from build123d import *

# Parameters (mm, degrees)
F2_R     = 19.05
F3_DEPTH = 25.4


with BuildPart() as f1:
    # F0 (on Right) → F1 (revolve)
    with BuildSketch(Plane.YZ):
        Polygon((-25.4, 16.811958), (0, 16.811958), (0, 26.336958), (0, 28.782088), (-6.35, 28.782088), (-6.35, 35.861958), (-25.4, 35.861958), align=None)
        Polygon((0, 26.336958), (0, 16.811958), (25.4, 16.811958), (25.4, 35.861958), (6.35, 35.861958), (6.35, 105.711958), (12.7, 105.711958), (12.7, 131.111958), (-12.7, 131.111958), (-12.7, 105.711958), (-6.35, 105.711958), (-6.35, 35.861958), (-6.35, 28.782088), (0, 28.782088), align=None)
    revolve(axis=Axis((0, 18.4531, 0), (0, 1, 0)))

    # F2 (on face) → F3 (cut)
    with BuildSketch(Plane.XZ.offset(6.35)):
        with BuildLine():
            ThreePointArc((19.05, 69.047159), (-13.470384, 82.517543), (0, 49.997159))
            ThreePointArc((0, 49.997159), (13.470384, 55.576775), (19.05, 69.047159))
        make_face()
        with Locations((69.047159, 0)):
            Circle(F2_R)
        with Locations((0, -69.047159)):
            Circle(F2_R)
        with Locations((-69.047159, 0)):
            Circle(F2_R)
    extrude(amount=-F3_DEPTH, mode=Mode.SUBTRACT)


solid = f1.part
Model file for the job. Use its own axes, mm. A direction names the side the tool comes from. Round coordinates to 2 decimals unless told otherwise and drop trailing zeros. Order: outer loops, then holes, each group sorted by start corner. A loop starts at its lowest first (then second) coordinate and runs counter-clockwise, first axis right, second up.
(1) Pin check, flat tips, straight feed: pin 1 (8 mm diameter, centred on y = -12, z = -79, fed in from +X); pin 2 (8 mm diameter, centred on x = 14.5, z = -42, fed in from -Y); pin 3 (1.5 mm diameter, centred on x = 92, y = 12, fed in from -Z); pin 4 (12 mm diameter, centred on x = 24.5, z = 27, fed in from -Y). Stop position of each tip, or through.
(2) Band-saw the part on C-C (y = 2). List the corners of the cut face in (x, z).
(3) Band-saw the part on D-D (z = 84.5). List the corners of the cut face in (x, y).
(4) Band-saw the part on B-B (x = 85). List the corners of the cut face in (y, z), then the cut area to 3 significant figures.
(5) 3-axis set-ups, long thin cutter, end or side, ignore diameter. For faces 1 (the face through (1, 6.35, -46)), 2 (the face through (35.557, -16.008, -4.669)), 3 (the face through (5.05, 0.356, 16.036)): which of +Z, -Z, +X, -X, +Y, -Y reach the whole face in a straight line?
(6) Drill centre lines: line 1 (X direction, y = 11.5, z = 1); line 2 (Z direction, x = -10, y = 9); line 3 (X direction, y = 11.25, z = 0). Where is each one in solid material? Low to high.
(7) Band-saw the part on A-A (z = 0). Give the number of separate pieces and of enclosed holes in the cut face, then the cut area to 3 significant figures.
(8) Pull direction Z, two halves, no side cores. Call faces 4 (the face through (-7.5, 25.4, -15.4)), 5 (the face through (129.996, -0.178, -17.068)), 6 (the face through (-51.45, -0.09, -7.3)): released by +Z, released by -Z, zero draft, split by the parting line, or undercut.
Verdict:
1. pin 1: stops at x = 107.54
1. pin 2: stops at y = -6.35
1. pin 3: stops at z = -94.15
1. pin 4: stops at y = -25.4
2. outline: circle Ø262.22 at (0, 0); hole circle Ø38.1 at (-69.05, 0); hole circle Ø38.1 at (0, -69.05); hole circle Ø38.1 at (0, 69.05); hole circle Ø33.62 at (0, 0); hole circle Ø38.1 at (69.05, 0)
3. outline: (-100.25, -12.7) - (-63.52, -12.7) - (-63.52, -6.35) - (-11.14, -6.35) - (-11.14, 6.35) - (-63.52, 6.35) - (-63.52, 12.7) - (-100.25, 12.7) - close; (11.14, -6.35) - (63.52, -6.35) - (63.52, -12.7) - (100.25, -12.7) - (100.25, 12.7) - (63.52, 12.7) - (63.52, 6.35) - (11.14, 6.35) - close
4. outline: (-12.7, -99.83) - (12.7, -99.83) - (12.7, -62.85) - (6.35, -62.85) - (6.35, -10.41) - (-6.35, -10.41) - (-6.35, -62.85) - (-12.7, -62.85) - close; (-12.7, 62.85) - (-6.35, 62.85) - (-6.35, 10.41) - (6.35, 10.41) - (6.35, 62.85) - (12.7, 62.85) - (12.7, 99.83) - (-12.7, 99.83) - close
4. area: 3,210 mm2
5. face 1: +Y
5. face 2: -Y
5. face 3: +Y, -Y
6. line 1: x = -131.11 to -105.71, -35.85 to -16.78, 16.78 to 35.85, 105.71 to 131.11
6. line 2: z = -130.73 to -105.24, -34.44 to -13.51, 13.51 to 34.44, 105.24 to 130.73
6. line 3: x = -131.11 to -105.71, -35.86 to -16.81, 16.81 to 35.86, 105.71 to 131.11
7. separate pieces: 4
7. enclosed holes: 0
7. area: 4,030 mm2
8. face 4: zero draft
8. face 5: split by the parting line
8. face 6: undercut
